Autodesk Fusion 360 part; units mm, degrees
sketch "Sketch1" plane through (0, 0, 0) normal (0, 1, 0) x (1, 0, 0)
  line L0 (-7.5, 7.625) -> (7.5, 7.625)
  line L1 (7.5, 7.625) -> (7.5, 4.625)
  line L2 (7.5, 4.625) -> (-7.5, 4.625)
  line L3 (-7.5, 4.625) -> (-7.5, 7.625)
  line L4 (-7.5, -4.625) -> (6.5, -4.625)
  line L5 (6.5, -4.625) -> (6.5, -7.625)
  line L6 (6.5, -7.625) -> (-7.5, -7.625)
  line L7 (-7.5, -7.625) -> (-7.5, -4.625)
  line L8 (-7.5, 7.625) -> (-9, 7.625)
  line L9 (-9, 7.625) -> (-9, -7.6278)
  line L10 (-9, -7.6278) -> (-7.5, -7.6278)
  line L11 (-7.5, -7.6278) -> (-7.5, 7.625)
  dimension "d3" = 4.625
  dimension "d4" = 4.625
  dimension "d5" = 15
  dimension "d6" = 7.5
  dimension "d7" = 14
  dimension "d9" = 7.5
  dimension "d10" = 1.5
extrude "Extrude1" add sketch "Sketch1" along normal blind 25
sketch "Sketch2" plane through (0, 0, -7.625) normal (0, 0, -1) x (-1, 0, 0)
  line L0 (-7.5, 0) -> (9, 0)
  line L1 (9, 0) -> (9, 25)
  line L2 (9, 25) -> (-7.5, 25)
  line L3 (-7.5, 25) -> (-7.5, 0)
  circle A0 centre (0, 12.5) radius 7
  dimension "d13" = 9
  dimension "d14" = 14
  dimension "d15" = 12.5
extrude "Extrude2" cut sketch "Sketch2" against normal blind 9 contours A0
equation "d3 = ( 9.25 / 2 ) * 1 mm"
equation "d4 = ( 9.25 / 2 ) * 1 mm"
The listing builds one solid part. Answer for the finished solid, in the listing's coordinates (mm). A direction names the side the tool comes from. Coordinates: 2 decimals unless noted, no trailing zeros. Write each loop counter-clockwise with the first axis right and the second up, starting at its lowest first coordinate (ties: lowest second). Pieces come first, ordered by that corner, then holes. Notation, with made-up numbers: (76.25, 64.5) - (124.25, 64.5) arc R9 ccw to (124.25, 70.5) - close; hole circle Ø6 at (26, 7). An arc over 180 degrees is marked (long way). Return JSON: item names as keys, results as strings. Group by question number.
Q1. Which of the six approach directions +Z, -Z, +X, -X, +Y, -Y give full straight-line access (tool end or side, diameter ignored) to faces 5 (the flat face through (6.5, 12, 6)), 6 (the flat face through (7.5, 12, -6)), 7 (the flat face through (-1, 12, 4.625))?
Q2. For a pull along Y with two mould halves and no side action, classify faces 1 (the flat face through (-8, 12, 7.628)), 2 (the flat face through (-1, 0, -5)), 3 (the flat face through (-1, 25, -5)), 4 (the cylindrical face through (1.517, 5.666, -6.146)) as +Y half, -Y half, draft (parallel to the pull), parting line (faces both ways), or undercut.
Q3. The part is cut by section C-C on z = 6.75. Write down the section's boundary in (x, y), and give its area (4 significant figures).
Q4. Find the intervals of material crossed by line 1 along Z through (x, y) = (-3.5, 2.25) (3 decimals); line 2 along Y through (x, z) = (0, -6.8); line 3 along Z through (x, y) = (0, 9.5) (3 decimals), in increasing order. Write a range as [from, to].
Q5. The part is cut by section B-B on x = 0. Write down the section's boundary in (y, z) (3 decimals).
Q6. Flat-ended cylindrical pins translate along their axes: pin 1 Ø1.5 at (y, z) = (9, 0) entering from +X; pin 2 Ø7.5 at (x, y) = (-1.5, 10.5) entering from +Z (3 decimals); pin 3 Ø0.9 at (y, z) = (9.5, 6) entering from +X. Find the tip coordinate at first contact, or state that the pin passes through.
Evaluation:
{
 "1": {"face 5": "+Z, +X, +Y, -Y", "face 6": "+Z, -Z, +X, +Y, -Y", "face 7": "+X, +Y, -Y"},
 "2": {"face 1": "draft", "face 2": "-Y half", "face 3": "+Y half", "face 4": "undercut"},
 "3": {"outline": "(-9, 0) - (6.5, 0) - (6.5, 25) - (-9, 25) - close", "area": "387.5 mm2"},
 "4": {"line 1": "z = [-7.625, -4.625], [4.625, 7.625]", "line 2": "y = [0, 5.5], [19.5, 25]", "line 3": "z = [4.625, 7.625]"},
 "5": {"outline": "(0, -7.625) - (5.5, -7.625) - (5.5, -4.625) - (0, -4.625) - close; (0, 4.625) - (25, 4.625) - (25, 7.625) - (0, 7.625) - close; (19.5, -7.625) - (25, -7.625) - (25, -4.625) - (19.5, -4.625) - close"},
 "6": {"pin 1": "stops at x = -7.5", "pin 2": "stops at z = 7.625", "pin 3": "stops at x = 6.5"}
}
